Geometry: see drawing. Coordinates: mm, zero at the bounding-box minimum. Coordinates: 2 decimals unless noted, no trailing zeros. Loops run counter-clockwise (first coordinate to the right, second up) from the corner with the lowest first, then second, coordinate; pieces in that order, holes last. Notation, with made-up numbers: (-0.5, 12) - (46.5, 12) arc R10 ccw to (46.5, 20) - close; hole circle Ø8 at (13.25, 31). An arc over 180 degrees is marked (long way). Write each question's results on one line, items separated by ' | '. Start each with the question number.
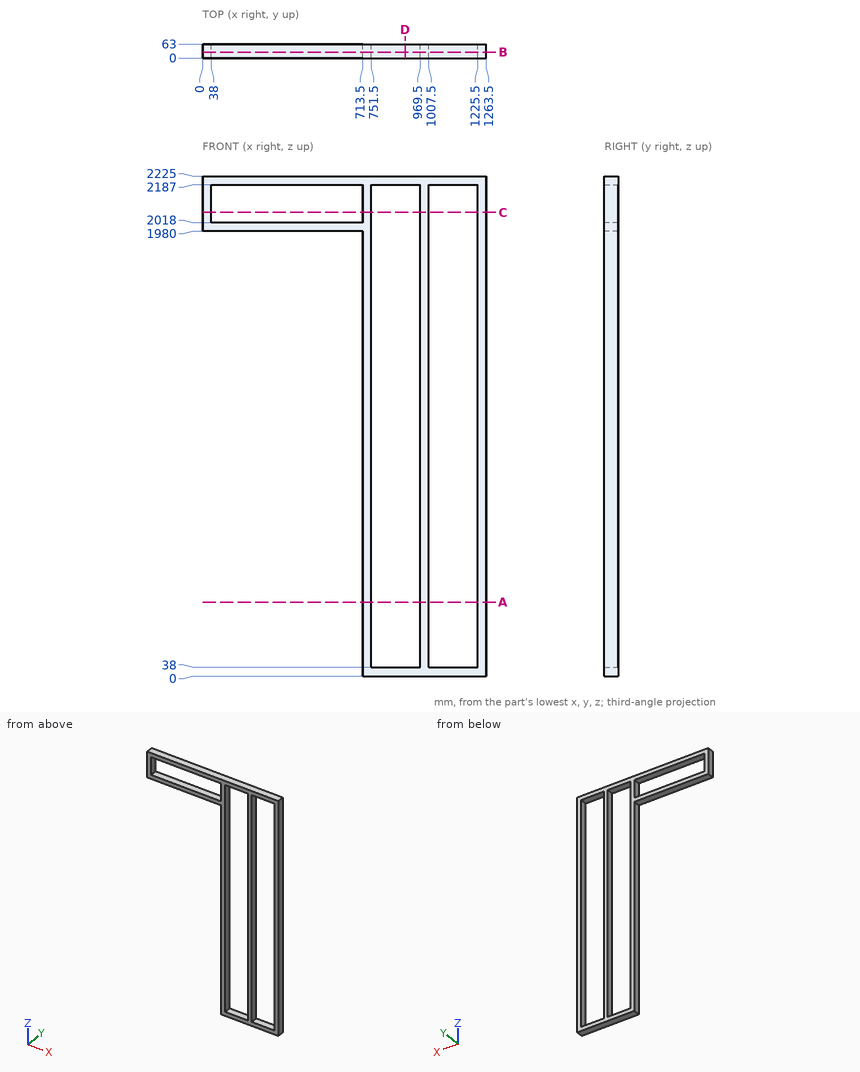
1) Section query D-D on x = 901.5. Output: boundary loops of the cut face in (y, z).
2) Pin query (flat end, axial travel): pin 1 Ø19 at (y, z) = (43, 1061) entering from -X; pin 2 Ø12 at (x, y) = (821, 31.5) entering from -Z. Return the tip coordinate at first contact, or that it passes through.
3) Section query B-B on y = 26.5. Output: boundary loops of the cut face in (x, z), and give its area (3 significant figures).
4) Material intervals for line 1 (X direction, y = 17.5, z = 1126); line 2 (X direction, y = 52.5, z = 2028.5); line 3 (Z direction, x = 1011.5, y = 35), sorted ascending. Write a range as [from, to].
5) Section query A-A on z = 329. Output: boundary loops of the cut face in (x, y), and give its area (3 significant figures).
6) Section query C-C on z = 2064. Output: boundary loops of the cut face in (x, y).
Returned:
1) outline: (0, 0) - (63, 0) - (63, 38) - (0, 38) - close; (0, 2187) - (63, 2187) - (63, 2225) - (0, 2225) - close
2) pin 1: stops at x = 713.5 | pin 2: stops at z = 0
3) outline: (0, 1980) - (713.5, 1980) - (713.5, 0) - (1263.5, 0) - (1263.5, 2225) - (0, 2225) - close; hole (38, 2018) - (713.5, 2018) - (713.5, 2187) - (38, 2187) - close; hole (751.5, 38) - (969.5, 38) - (969.5, 2187) - (751.5, 2187) - close; hole (1007.5, 38) - (1225.5, 38) - (1225.5, 2187) - (1007.5, 2187) - close | area: 347,000 mm²
4) line 1: x = [713.5, 751.5], [969.5, 1007.5], [1225.5, 1263.5] | line 2: x = [0, 38], [713.5, 751.5], [969.5, 1007.5], [1225.5, 1263.5] | line 3: z = [0, 38], [2187, 2225]
5) outline: (713.5, 0) - (751.5, 0) - (751.5, 63) - (713.5, 63) - close; (969.5, 0) - (1007.5, 0) - (1007.5, 63) - (969.5, 63) - close; (1225.5, 0) - (1263.5, 0) - (1263.5, 63) - (1225.5, 63) - close | area: 7,180 mm²
6) outline: (0, 0) - (38, 0) - (38, 63) - (0, 63) - close; (713.5, 0) - (751.5, 0) - (751.5, 63) - (713.5, 63) - close; (969.5, 0) - (1007.5, 0) - (1007.5, 63) - (969.5, 63) - close; (1225.5, 0) - (1263.5, 0) - (1263.5, 63) - (1225.5, 63) - close
